For this review, take the finished solid that the model builds, in its own axes (mm). A direction names the side the tool comes from. Round coordinates to 2 decimals unless told otherwise and drop trailing zeros. Write each loop counter-clockwise with the first axis right and the second up, starting at its lowest first coordinate (ties: lowest second). Pieces come first, ordered by that corner, then holes. Notation, with made-up numbers: M 39,40 L 57,40 A27 ccw 57,71 Z; hole C 5,67.5 d2. An arc over 180 degrees is marked long. Use one line per item in the form item = value. Start each with the question number.
Item 1: Add section C-C (z = 0). State the section outline as (x, y) points (3 decimals), and give its area (3 significant figures).
Item 2: For P1, Ø8, axis at y = 87.5, z = -55, coming from the +X side; P2, Ø2, axis at x = 13.5, y = 346, coming from the -Z side; P3, Ø5, axis at x = 42, z = -63, coming from the +Y side, all flat-tipped, find the tip position at first contact; note any pin that passes through.
Item 3: Draft analysis for pull direction Z (two halves, no side actions). For faces 1 (the cylindrical face through (-15.497, 488.08, -3.441)), 2 (the flat face through (-3, 495.3, -4)), 3 (the cylindrical face through (-2.951, 487.176, 3.873)), state which applies: released by +Z, released by -Z, zero draft, split by the parting line, or undercut.
Item 4: Add section B-B (z = -43.5). State the section outline as (x, y) points.
Item 5: Add section A-A (x = 51.5). State the section outline as (y, z) points, and give its area (3 significant figures).
Item 6: Add section D-D (y = 447.5). State the section outline as (x, z) points, and give its area (3 significant figures).
Item 7: For faces 4 (the cylindrical face through (-17.895, 239.078, 80.587)), 5 (the cylindrical face through (75.71, 243.52, -23.84)), list the 3-axis set-ups (+Z, -Z, +X, -X, +Y, -Y) from which the entire face can be reached by the end or side of a thin tool; tool diameter is ignored.
Item 8: For line 1 (Z direction, x = 0, y = 160) (3 decimals); line 2 (Z direction, x = 25, y = 219), list the stretches that pass through material, from the lowest coordinate up. Write a range as [from, to].
from build123d import *

# Parameters (mm, degrees)
BOSS_EXTRUDE1_REACH              = 498.52
BOSS_EXTRUDE1_END_RADIUS         = 82.55
SKETCH2_R                        = 15.875
BOSS_EXTRUDE1_DIRECTION_2_DEPTH  = 12.7
F_3_8_0_375_DIAMETER_HOLE1_D     = 9.525
F_3_8_0_375_DIAMETER_HOLE1_DEPTH = 25.4
F_3_8_0_375_DIAMETER_HOLE1_TIP   = 2.861598698


with BuildPart() as part:
    # Sketch1 → Revolve1 (revolve)
    with BuildSketch(Plane.XY):
        with BuildLine():
            Line((82.55, 400.05), (82.55, 82.55))
            ThreePointArc((82.55, 82.55), (58.371664787, 24.178335213), (0, 0))
            Line((0, 0), (0, 3.175))
            ThreePointArc((0, 3.175), (56.126600757, 26.423399243), (79.375, 82.55))
            Line((79.375, 82.55), (79.375, 400.05))
            ThreePointArc((79.375, 400.05), (56.126600757, 456.176600757), (0, 479.425))
            Line((0, 479.425), (0, 482.6))
            ThreePointArc((0, 482.6), (58.371664787, 458.421664787), (82.55, 400.05))
        make_face()
    revolve(axis=Axis((0, 482.6, 0), (0, 1, 0)))

    # Boss-Extrude1: up to this sphere (the profile starts outside it)
    boss_extrude1_end = Location((0, 400.05, 0)) * Sphere(BOSS_EXTRUDE1_END_RADIUS, mode=Mode.PRIVATE)
    # Sketch2 → Boss-Extrude1 (add, up to the surface)
    with BuildSketch(Plane(origin=(0, 482.6, 0), x_dir=(1, 0, 0), z_dir=(0, 1, 0)), mode=Mode.PRIVATE) as boss_extrude1_sk1:
        with Locations(Location((0, 0, 0), (0, 0, 270))):
            Circle(SKETCH2_R)
    boss_extrude1_tool1 = extrude(boss_extrude1_sk1.sketch, amount=-BOSS_EXTRUDE1_REACH, mode=Mode.PRIVATE) - boss_extrude1_end
    add(boss_extrude1_tool1.solids().sort_by_distance((0, 482.6, 0))[0])

    # Sketch2 → Boss-Extrude1 direction 2 (add)
    with BuildSketch(Plane(origin=(0, 482.6, 0), x_dir=(1, 0, 0), z_dir=(0, 1, 0))):
        with Locations(Location((0, 0, 0), (0, 0, 270))):
            Circle(SKETCH2_R)
    extrude(amount=BOSS_EXTRUDE1_DIRECTION_2_DEPTH)

    # 3/8 (0.375) Diameter Hole1
    with Locations(Plane(origin=(-0.053238661, 495.3, 0.09377676), x_dir=(0, 0, 1), z_dir=(0, 1, 0))):
        with Locations((0, 0)):
            Hole(F_3_8_0_375_DIAMETER_HOLE1_D / 2, depth=F_3_8_0_375_DIAMETER_HOLE1_DEPTH)
            with Locations((0, 0, -(F_3_8_0_375_DIAMETER_HOLE1_DEPTH + F_3_8_0_375_DIAMETER_HOLE1_TIP / 2))):  # 118° drill point
                Cone(0, F_3_8_0_375_DIAMETER_HOLE1_D / 2, F_3_8_0_375_DIAMETER_HOLE1_TIP, mode=Mode.SUBTRACT)


solid = part.part
Calculated:
q1.outline = M -82.55,82.55 A82.55 ccw 82.55,82.55 L 82.55,400.05 A82.55 ccw 15.875,481.059 L 15.875,495.3 L 4.708,495.3 L 4.708,479.285 A79.375 cw 79.375,400.05 L 79.375,82.55 A79.375 cw -79.375,82.55 L -79.375,400.05 A79.375 cw -4.815,479.279 L -4.815,495.3 L -15.875,495.3 L -15.875,481.059 A82.55 ccw -82.55,400.05 Z
q1.area = 3,900 mm^2
q2.P1 = 64.91
q2.P2 = -81.6
q2.P3 = 438.18
q3.face_1 = split by the parting line
q3.face_2 = zero draft
q3.face_3 = undercut
q4.outline = M -70.16,82.55 A70.16 ccw 70.16,82.55 L 70.16,400.05 A70.16 ccw -70.16,400.05 Z; hole M -66.39,82.55 A66.39 ccw 66.39,82.55 L 66.39,400.05 A66.39 ccw -66.39,400.05 Z
q5.outline = M 82.55,-64.52 L 400.05,-64.52 A64.52 ccw 400.05,64.52 L 82.55,64.52 A64.52 ccw Z; hole M 82.55,-60.4 L 400.05,-60.4 A60.4 ccw 400.05,60.4 L 82.55,60.4 A60.4 ccw Z
q5.area = 4,230 mm^2
q6.outline = C 0,0 d135.1; hole C 0,0 d127.26
q6.area = 1,620 mm^2
q7.face_4 = +Y, -Y
q7.face_5 = none
q8.line_1 = [-82.55, -79.375], [79.375, 82.55]
q8.line_2 = [-78.67, -75.34], [75.34, 78.67]
